Design review of the part built by this model. Coordinates are the model's own, in mm. A direction names the side the tool comes from. Round coordinates to 2 decimals unless told otherwise and drop trailing zeros. Loops run counter-clockwise (first coordinate to the right, second up) from the corner with the lowest first, then second, coordinate; pieces in that order, holes last. Notation, with made-up numbers: M 46,51.5 L 59,51.5 A35 ccw 59,85.5 Z; hole C -35.75,36 d10. An arc over 180 degrees is marked long. One line per item, written item: value. Start each with the question number.
Item 1: We need section D-D (x = -6.5). Write out the cut boundary in (y, z).
Item 2: We need section C-C (z = 17.75). Write out the cut boundary in (x, y).
Item 3: Mouldability with a two-part tool opening along X and no side actions: class faces 4 (the cylindrical face through (-24.98, -7.34, 9.54)), 5 (the flat face through (20, 4, 10)), 6 (the flat face through (-21, -8.864, 10)), 7 (the cylindrical face through (25.016, -7.343, 9.676)) as released by +X, released by -X, zero draft, split by the parting line, or undercut.
Item 4: We need section B-B (x = 0). Write out the cut boundary in (y, z), then the cut area to 3 significant figures.
Item 5: For line 1 along X through (y, z) = (-7.05, 10); line 2 along X through (y, z) = (0, 15.75); line 3 along Z through (x, y) = (23.5, -7.8), list the stretches that pass through material, from the lowest coordinate up.
Item 6: We need section A-A (y = 1.75). Write out the cut boundary in (x, z), then the cut area to 3 significant figures.
Item 7: For faces 1 (the flat face through (25.3, -5.864, 9.9)), 2 (the flat face through (0, 12.136, 5)), 3 (the cylindrical face through (-16.43, 8.534, 10.14)), list the 3-axis set-ups (+Z, -Z, +X, -X, +Y, -Y) from which the entire face can be reached by the end or side of a thin tool; tool diameter is ignored.
Item 8: Clearance check with flat-ended pins moving along their axes: pin 1 (4 mm diameter, centred on y = -1, z = 4, fed in from +X); pin 2 (1 mm diameter, centred on y = 3, z = 6, fed in from -X); pin 3 (6.5 mm diameter, centred on x = 0, z = 10, fed in from +Y); pin 4 (4.5 mm diameter, centred on x = 23.5, z = 10, fed in from +Y). State where each tip first meets the part, or that it passes through.
from build123d import *

# Parameters (mm, degrees)
BOSS_EXTRUDE1_DEPTH = 20
SKETCH2_R           = 4.05
CUT_EXTRUDE1_DEPTH  = 16
FILLET1_R           = 2
SKETCH3_R           = 1.55
CUT_EXTRUDE2_DEPTH  = 16


with BuildPart() as part:
    # Sketch1 → Boss-Extrude1 (new body)
    with BuildSketch(Plane.XY):
        Polygon((-17, -8.864115169), (-26, -8.864115169), (-26, -5.864115169), (-20, -5.864115169), (-20, 12.135884831), (20, 12.135884831), (20, -5.864115169), (26, -5.864115169), (26, -8.864115169), (17, -8.864115169), (17, 9.135884831), (-17, 9.135884831), align=None)
    extrude(amount=BOSS_EXTRUDE1_DEPTH)

    # Sketch2 → Cut-Extrude1 (cut)
    with BuildSketch(Plane(origin=(0, 12.135884831, 0), x_dir=(1, 0, 0), z_dir=(0, 1, 0))):
        with Locations(Location((0, -10, 0), (0, 0, 270))):
            Circle(SKETCH2_R)
    extrude(amount=-CUT_EXTRUDE1_DEPTH, mode=Mode.SUBTRACT)

    # Fillet1
    fillet1_edges = [part.edges().sort_by_distance(p)[0] for p in [
        (-20, -5.864115169, 10),
        (20, -5.864115169, 10),
        (17, 9.135884831, 10),
        (-17, 9.135884831, 10),
    ]]
    fillet(fillet1_edges, radius=FILLET1_R)

    # Sketch3 → Cut-Extrude2 (cut)
    with BuildSketch(Plane(origin=(0, -5.864115169, 0), x_dir=(1, 0, 0), z_dir=(0, 1, 0))):
        with Locations(Location((-23.5, -10, 0), (0, 0, 345.407449398))):
            Circle(SKETCH3_R)
        with Locations(Location((23.5, -10, 0), (0, 0, 194.592550602))):
            Circle(SKETCH3_R)
    extrude(amount=-CUT_EXTRUDE2_DEPTH, mode=Mode.SUBTRACT)


solid = part.part
A:
1. outline: M 9.14,0 L 12.14,0 L 12.14,20 L 9.14,20 Z
2. outline: M -26,-8.86 L -17,-8.86 L -17,7.14 A2 cw -15,9.14 L 15,9.14 A2 cw 17,7.14 L 17,-8.86 L 26,-8.86 L 26,-5.86 L 22,-5.86 A2 cw 20,-3.86 L 20,12.14 L -20,12.14 L -20,-3.86 A2 cw -22,-5.86 L -26,-5.86 Z
3. face 4: undercut
3. face 5: released by +X
3. face 6: zero draft
3. face 7: undercut
4. outline: M 9.14,0 L 12.14,0 L 12.14,5.95 L 9.14,5.95 Z; M 9.14,14.05 L 12.14,14.05 L 12.14,20 L 9.14,20 Z
4. area: 35.7 mm2
5. line 1: -26 to -25.05, -21.95 to -17, 17 to 21.95, 25.05 to 26
5. line 2: -20 to -17, 17 to 20
5. line 3: 0 to 8.45, 11.55 to 20
6. outline: M -20,0 L -17,0 L -17,20 L -20,20 Z; M 17,0 L 20,0 L 20,20 L 17,20 Z
6. area: 120 mm2
7. face 1: +Z, -Z, +X, +Y
7. face 2: +Z, -Z, +X, -X, +Y
7. face 3: +Z, -Z, -Y
8. pin 1: x = 20
8. pin 2: x = -20
8. pin 3: through
8. pin 4: y = -5.72
